Autodesk Inventor part; units mm, degrees
ref_plane "YZ Plane" through (0, 0, 0) normal (1, 0, 0) x (0, 1, 0)
ref_plane "XZ Plane" through (0, 0, 0) normal (0, 1, 0) x (-1, 0, 0)
ref_plane "XY Plane" through (0, 0, 0) normal (0, 0, 1) x (1, 0, 0)
sketch "Sketch1" plane through (0, 0, 0) normal (0, 1, 0) x (-1, 0, 0)
  line L0 (0, 0) -> (69.85, 0)
  line L1 (69.85, 0) -> (69.85, -355.6)
  line L2 (69.85, -355.6) -> (0, -355.6)
  line L3 (0, -355.6) -> (0, 0)
  dimension "d0" = 69.85
  dimension "d1" = 355.6
extrude "Extrusion1" add sketch "Sketch1" along normal blind 44.45
fillet "Fillet1" radius 14.2875 4 edges at (0, 22.225, 0) (-69.85, 22.225, 0) (0, 22.225, -355.6) (-69.85, 22.225, -355.6)
sketch "Sketch3" plane through (0, 44.45, 0) normal (0, 1, 0) x (1, 0, 0)
  arc A0 (-55.5625, 355.6) -> (-69.85, 341.3125) centre (-55.5625, 341.3125) ccw
  line L0 (-69.85, 341.3125) -> (-69.85, 14.2875)
  arc A1 (-69.85, 14.2875) -> (-55.5625, 0) centre (-55.5625, 14.2875) ccw
  line L1 (-55.5625, 0) -> (-14.2875, 0)
  arc A2 (-14.2875, 0) -> (0, 14.2875) centre (-14.2875, 14.2875) ccw
  line L2 (0, 14.2875) -> (0, 341.3125)
  arc A3 (0, 341.3125) -> (-14.2875, 355.6) centre (-14.2875, 341.3125) ccw
  line L3 (-14.2875, 355.6) -> (-55.5625, 355.6)
  line L4 (-19.685, 333.0203) -> (-50.165, 333.0203)
  line L5 (-50.165, 333.0203) -> (-50.165, 319.6698)
  line L6 (-50.165, 319.6698) -> (-19.685, 319.6698)
  line L7 (-19.685, 319.6698) -> (-19.685, 333.0203)
  line L8 (-19.685, 333.0203) -> (-50.165, 319.6698) construction
  line L9 (-50.165, 333.0203) -> (-19.685, 319.6698) construction
  point P0 (0, 0)
  point P1 (-34.925, 326.345)
extrude "Extrusion3" add sketch "Sketch3" along normal blind 3.175 contours L7 L6 L5 L4
properties part number "power strip"
Read the model definition and answer for the solid it produces. Units are mm, in the model's axes. Round coordinates to 2 decimals unless told otherwise and drop trailing zeros. Order: outer loops, then holes, each group sorted by start corner. A loop starts at its lowest first (then second) coordinate and runs counter-clockwise, first axis right, second up.
1) The part is cut by section C-C on x = -60. Write down the section's boundary in (y, z).
2) Straight lines are drawn through the part: L1, parallel to Y at x = -29.5, z = -76; L2, parallel to Z at x = -35.5, y = 46; L3, parallel to Z at x = -7, y = 22. For each, find the intervals that lie inside material, in ascending order.
3) The part is cut by section A-A on x = -45. Write down the section's boundary in (y, z) (3 decimals).
4) Flat-ended cylindrical pins translate along their axes: pin 1 (2 mm diameter, centred on x = -49.5, z = -177.5, fed in from +Y); pin 2 (1 mm diameter, centred on x = -13, y = 41, fed in from -Z); pin 3 (2.5 mm diameter, centred on x = -41, y = 46, fed in from +Z). Find the tip coordinate at first contact, or state that the pin passes through.
5) The part is cut by section B-B on z = -29. Write down the section's boundary in (x, y).
Resolved:
1. outline: (0, -354.89) - (44.45, -354.89) - (44.45, -0.71) - (0, -0.71) - close
2. L1: y = 0 to 44.45
2. L2: z = -333.02 to -319.67
2. L3: z = -353.6 to -2
3. outline: (0, -355.6) - (44.45, -355.6) - (44.45, -333.02) - (47.625, -333.02) - (47.625, -319.67) - (44.45, -319.67) - (44.45, 0) - (0, 0) - close
4. pin 1: stops at y = 44.45
4. pin 2: stops at z = -355.58
4. pin 3: stops at z = -319.67
5. outline: (-69.85, 0) - (0, 0) - (0, 44.45) - (-69.85, 44.45) - close
